Autodesk Inventor part; units mm, degrees
ref_plane "YZ Plane" through (0, 0, 0) normal (1, 0, 0) x (0, 1, 0)
ref_plane "XZ Plane" through (0, 0, 0) normal (0, 1, 0) x (-1, 0, 0)
ref_plane "XY Plane" through (0, 0, 0) normal (0, 0, 1) x (1, 0, 0)
sketch "Sketch1" plane through (0, 0, 0) normal (0, 1, 0) x (-1, 0, 0)
  circle A0 centre (15.5, 15.5) radius 1.5
  circle A1 centre (15.5, -15.5) radius 1.5
  circle A2 centre (-15.5, -15.5) radius 1.5
  circle A3 centre (-15.5, 15.5) radius 1.5
  circle A4 centre (0, 0) radius 11
  circle A5 centre (0, 0) radius 4
  line L0 (21, -17) -> (17, -21)
  line L1 (21, 17) -> (17, 21)
  line L2 (-17, -21) -> (-21, -17)
  line L3 (-21, 17) -> (-17, 21)
  circle A6 centre (0, 0) radius 2.5
  line L4 (17, -21) -> (-17, -21)
  line L5 (-21, -17) -> (-21, 17)
  line L6 (-17, 21) -> (17, 21)
  line L7 (21, 17) -> (21, -17)
  line L8 (0, -15.5) -> (-15.5, -15.5) construction
  line L9 (0, -15.5) -> (15.5, -15.5) construction
  line L10 (15.5, -15.5) -> (15.5, 15.5) construction
  line L11 (-15.5, -15.5) -> (-15.5, 15.5) construction
  line L12 (0, -21) -> (0, 0) construction
  line L13 (0, 0) -> (21, 0) construction
  point P0 (0, 0)
  dimension "d0" = 31
  dimension "d1" = 31
  dimension "d2" = 31
  dimension "d3" = 31
  dimension "d4" = 3
  dimension "d5" = 3
  dimension "d6" = 3
  dimension "d7" = 3
  dimension "d8" = 22
  dimension "d9" = 8
  dimension "d10" = 5
  dimension "d11" = 15.5
  dimension "d12" = 42
  dimension "d13" = 42
  dimension "d14" = 15.5
  dimension "d15" = 21
  dimension "d16" = 21
  dimension "d17" = 34
  dimension "d18" = 34
  dimension "d19" = 135
sketch "Sketch2" plane through (0, 0, 0) normal (0, 1, 0) x (-1, 0, 0)
  line L0 (-15.5, 15.5) -> (15.5, 15.5) construction
  line L1 (15.5, 15.5) -> (15.5, -15.5) construction
  line L2 (15.5, -15.5) -> (-15.5, -15.5) construction
  line L3 (-15.5, -15.5) -> (-15.5, 15.5) construction
  line L4 (-15.5, 15.5) -> (15.5, -15.5) construction
  line L5 (15.5, 15.5) -> (-15.5, -15.5) construction
  circle A0 centre (-15.5, -15.5) radius 1.6
  circle A1 centre (15.5, -15.5) radius 1.6
  circle A2 centre (15.5, 15.5) radius 1.6
  circle A3 centre (-15.5, 15.5) radius 1.6
  line L6 (21, -17) -> (17, -21)
  line L7 (21, -17) -> (21, 17)
  line L8 (21, 17) -> (17, 21)
  line L9 (17, 21) -> (-17, 21)
  line L10 (-17, 21) -> (-21, 17)
  line L11 (-21, 17) -> (-21, -17)
  line L12 (-21, -17) -> (-17, -21)
  line L13 (-17, -21) -> (17, -21)
  line L14 (0, -21) -> (0, -15.5) construction
  line L15 (0, 15.5) -> (0, 21) construction
  line L16 (-15.5, 0) -> (-21, 0) construction
  line L17 (15.5, 0) -> (21, 0) construction
  line L18 (-24, -24) -> (37.7656, -24)
  line L19 (37.7656, -24) -> (37.7656, 24)
  line L20 (37.7656, 24) -> (-24, 24)
  line L21 (-24, 24) -> (-24, -24)
  line L22 (-24, 20) -> (-18, 20)
  line L23 (-24, -20) -> (-18, -20)
  line L24 (-18, 20) -> (-18, 24) construction
  line L25 (-18, -20) -> (-18, -24) construction
  point P0 (0, 0)
  dimension "d20" = 31
  dimension "d22" = 3.2
  dimension "d23" = 135
  dimension "d24" = 42
  dimension "d25" = 34
  dimension "d33" = 3
  dimension "d34" = 3
  dimension "d35" = 3
  dimension "d37" = 40
sketch "Sketch3" plane through (0, 0, 0) normal (0, 1, 0) x (-1, 0, 0)
  line L0 (29.4, -16) -> (29.4, 16) construction
  circle A0 centre (29.4, -16) radius 2.7
  circle A1 centre (29.4, 16) radius 2.7
  line L1 (0, 0) -> (29.4, 0)
  dimension "d30" = 32
  dimension "d31" = 5.4
  dimension "d32" = 29.4
extrude "Extrusion1" add sketch "Sketch2" along normal blind 10 contours L7 L8 L9 L10 L22 L21 L20 L19 L18 L23 L12 L13 L6
extrude "Extrusion2" cut sketch "Sketch3" along normal through all
equation "\"d1\" = d0"
equation "\"d2\" = d0"
equation "\"d3\" = d0"
equation "\"d5\" = d4"
equation "\"d6\" = d4"
equation "\"d7\" = d4"
equation "\"d11\" = 0.5 * d0"
equation "\"d13\" = d12"
equation "\"d15\" = 0.5 * d12"
equation "\"d16\" = 0.5 * d13"
equation "\"d34\" = d33"
properties part number "Stepper Z Mount"
Here's how the part is built. I have some questions about the finished solid (model axes, mm). A direction names the side the tool comes from. Give positions to 0.01 mm unless a question says otherwise; leave off trailing zeros. Loops run counter-clockwise (first coordinate to the right, second up) from the corner with the lowest first, then second, coordinate; pieces in that order, holes last. Notation, with made-up numbers: (-31, -37.75) -> (-7, -37.75) arc R15 cw to (-7, -33.75) -> close; hole circle Ø8 at (18, 34.25). An arc over 180 degrees is marked (long way). Use one line per item in the form item = value. Start each with the question number.
1) Imagine slicing it at A-A (z = 16). Please give me the cut outline in (x, y).
2) Imagine slicing it at B-B (x = -1.5). Please give me the cut outline in (y, z).
3) Imagine slicing it at D-D (x = -29.4). Please give me the cut outline in (y, z).
4) Thinking about a two-plate mould opening in X: for faces 1 (the face through (-21, 5, 0)), 2 (the face through (-31.975, 4.93, 15.189)), 3 (the face through (-6, 5, -24)), which applies, +X half, -X half, draft (parallel to the pull), parting line (faces both ways), or undercut?
5) Please list where these lines run through material, in increasing order: line 1 along Z through (x, y) = (-29.4, 7.5); line 2 along X through (y, z) = (4.25, 16); line 3 along Z through (x, y) = (0, 9.5).
6) For P1, Ø3, axis at x = -29.4, z = -16, coming from the +Y side; P2, Ø2, axis at y = 4, z = 8.5, coming from the +X side, each with a flat end and sliding along its axis, tell me the tip position at first contact or that it passes through.
7) Which directions (+Z, -Z, +X, -X, +Y, -Y) give clear straight access to the entire face, cutting with the end or side of a thin tool? Please do faces 4 (the face through (-19, 5, 19)), 5 (the face through (24, 5, 22)), 6 (the face through (21, 5, -20)).
8) Imagine slicing it at C-C (y = 3.5). Please give me the cut outline in (x, z).
Check values:
q1.outline = (-37.77, 0) -> (-32.1, 0) -> (-32.1, 10) -> (-37.77, 10) -> close; (-26.7, 0) -> (-21, 0) -> (-21, 10) -> (-26.7, 10) -> close
q2.outline = (0, -24) -> (10, -24) -> (10, -21) -> (0, -21) -> close; (0, 21) -> (10, 21) -> (10, 24) -> (0, 24) -> close
q3.outline = (0, -24) -> (10, -24) -> (10, -18.7) -> (0, -18.7) -> close; (0, -13.3) -> (10, -13.3) -> (10, 13.3) -> (0, 13.3) -> close; (0, 18.7) -> (10, 18.7) -> (10, 24) -> (0, 24) -> close
q4.face_1 = +X half
q4.face_2 = undercut
q4.face_3 = draft
q5.line_1 = -24 to -18.7, -13.3 to 13.3, 18.7 to 24
q5.line_2 = -37.77 to -32.1, -26.7 to -21
q5.line_3 = -24 to -21, 21 to 24
q6.P1 = through
q6.P2 = -21
q7.face_4 = +Y, -Y
q7.face_5 = +Z, -Z, +X, +Y, -Y
q7.face_6 = +X, +Y, -Y
q8.outline = (-37.77, -24) -> (24, -24) -> (24, -20) -> (18, -20) -> (17, -21) -> (-17, -21) -> (-21, -17) -> (-21, 17) -> (-17, 21) -> (17, 21) -> (18, 20) -> (24, 20) -> (24, 24) -> (-37.77, 24) -> close; hole circle Ø5.4 at (-29.4, -16); hole circle Ø5.4 at (-29.4, 16)
